```python
from build123d import *

# Parameters (mm, degrees)
BOSS_EXTRUDE1_DEPTH = 2
BOSS_EXTRUDE2_DEPTH = 60
CUT_EXTRUDE1_REACH  = 109.268
SKETCH2_R           = 11
SKETCH2_R_2         = 2.75
SKETCH3_R           = 2
CUT_EXTRUDE2_DEPTH  = 3
FILLET1_R           = 4


with BuildPart() as part:
    # Sketch1 → Boss-Extrude1 (new body)
    with BuildSketch(Plane(origin=(0, 0, 0), x_dir=(0, 0, -1), z_dir=(1, 0, 0))):
        Polygon((12.587763003, 38.086063364), (80, 3), (3.839824897, 3), align=None)
        Polygon((9.676875824, 38.811829051), (12.587763003, 38.086063364), (3.839824897, 3), (80, 3), (80, 0), (0, 0), align=None)
    extrude(amount=-BOSS_EXTRUDE1_DEPTH)

    # Sketch1<3> → Boss-Extrude2 (add)
    with BuildSketch(Plane(origin=(0, 0, 0), x_dir=(0, 0, -1), z_dir=(1, 0, 0))):
        Polygon((9.676875824, 38.811829051), (12.587763003, 38.086063364), (3.839824897, 3), (80, 3), (80, 0), (0, 0), align=None)
    extrude(amount=-BOSS_EXTRUDE2_DEPTH)

    # Sketch2 → Cut-Extrude1 (cut, up to next)
    with BuildSketch(Plane(origin=(0, 0, 0), x_dir=(1, 0, 0), z_dir=(0, 0.24192189559967164, 0.9702957262759956)), mode=Mode.PRIVATE) as cut_extrude1_sk1:
        with Locations(Location((-30, 20, 0), (0, 0, 270))):
            Circle(SKETCH2_R)
    cut_extrude1_tool1 = extrude(cut_extrude1_sk1.sketch, amount=-CUT_EXTRUDE1_REACH, mode=Mode.PRIVATE) & part.part
    # Sketch2 → Cut-Extrude1 (cut, up to next)
    with BuildSketch(Plane(origin=(0, 0, 0), x_dir=(1, 0, 0), z_dir=(0, 0.24192189559967164, 0.9702957262759956)), mode=Mode.PRIVATE) as cut_extrude1_sk2:
        with Locations(Location((-50, 20, 0), (0, 0, 270))):
            Circle(SKETCH2_R_2)
    cut_extrude1_tool2 = extrude(cut_extrude1_sk2.sketch, amount=-CUT_EXTRUDE1_REACH, mode=Mode.PRIVATE) & part.part
    # Sketch2 → Cut-Extrude1 (cut, up to next)
    with BuildSketch(Plane(origin=(0, 0, 0), x_dir=(1, 0, 0), z_dir=(0, 0.24192189559967164, 0.9702957262759956)), mode=Mode.PRIVATE) as cut_extrude1_sk3:
        with Locations(Location((-10, 20, 0), (0, 0, 90))):
            Circle(SKETCH2_R_2)
    cut_extrude1_tool3 = extrude(cut_extrude1_sk3.sketch, amount=-CUT_EXTRUDE1_REACH, mode=Mode.PRIVATE) & part.part
    add(cut_extrude1_tool1.solids().sort_by_distance((-30, 19.405915, -4.838438))[0], mode=Mode.SUBTRACT)
    add(cut_extrude1_tool2.solids().sort_by_distance((-50, 19.405915, -4.838438))[0], mode=Mode.SUBTRACT)
    add(cut_extrude1_tool3.solids().sort_by_distance((-10, 19.405915, -4.838438))[0], mode=Mode.SUBTRACT)

    # Sketch3 → Cut-Extrude2 (cut)
    with BuildSketch(Plane.XZ):
        with Locations(Location((-55, -33, 0), (0, 0, 270))):
            Circle(SKETCH3_R)
        with Locations(Location((-47, -33, 0), (0, 0, 270))):
            Circle(SKETCH3_R)
        with Locations(Location((-39, -33, 0), (0, 0, 270))):
            Circle(SKETCH3_R)
        with Locations(Location((-31, -33, 0), (0, 0, 270))):
            Circle(SKETCH3_R)
        with Locations(Location((-23, -33, 0), (0, 0, 270))):
            Circle(SKETCH3_R)
        with Locations(Location((-15, -33, 0), (0, 0, 270))):
            Circle(SKETCH3_R)
        with Locations(Location((-47, -41, 0), (0, 0, 270))):
            Circle(SKETCH3_R)
        with Locations(Location((-39, -41, 0), (0, 0, 270))):
            Circle(SKETCH3_R)
        with Locations(Location((-31, -41, 0), (0, 0, 270))):
            Circle(SKETCH3_R)
        with Locations(Location((-23, -41, 0), (0, 0, 270))):
            Circle(SKETCH3_R)
        with Locations(Location((-15, -41, 0), (0, 0, 270))):
            Circle(SKETCH3_R)
        with Locations(Location((-47, -49, 0), (0, 0, 270))):
            Circle(SKETCH3_R)
        with Locations(Location((-39, -49, 0), (0, 0, 270))):
            Circle(SKETCH3_R)
        with Locations(Location((-31, -49, 0), (0, 0, 270))):
            Circle(SKETCH3_R)
        with Locations(Location((-23, -49, 0), (0, 0, 270))):
            Circle(SKETCH3_R)
        with Locations(Location((-15, -49, 0), (0, 0, 270))):
            Circle(SKETCH3_R)
        with Locations(Location((-47, -57, 0), (0, 0, 270))):
            Circle(SKETCH3_R)
        with Locations(Location((-39, -57, 0), (0, 0, 270))):
            Circle(SKETCH3_R)
        with Locations(Location((-31, -57, 0), (0, 0, 270))):
            Circle(SKETCH3_R)
        with Locations(Location((-23, -57, 0), (0, 0, 270))):
            Circle(SKETCH3_R)
        with Locations(Location((-15, -57, 0), (0, 0, 270))):
            Circle(SKETCH3_R)
        with Locations(Location((-47, -65, 0), (0, 0, 270))):
            Circle(SKETCH3_R)
        with Locations(Location((-39, -65, 0), (0, 0, 270))):
            Circle(SKETCH3_R)
        with Locations(Location((-31, -65, 0), (0, 0, 270))):
            Circle(SKETCH3_R)
        with Locations(Location((-23, -65, 0), (0, 0, 270))):
            Circle(SKETCH3_R)
        with Locations(Location((-15, -65, 0), (0, 0, 270))):
            Circle(SKETCH3_R)
        with Locations(Location((-47, -73, 0), (0, 0, 270))):
            Circle(SKETCH3_R)
        with Locations(Location((-39, -73, 0), (0, 0, 270))):
            Circle(SKETCH3_R)
        with Locations(Location((-31, -73, 0), (0, 0, 270))):
            Circle(SKETCH3_R)
        with Locations(Location((-23, -73, 0), (0, 0, 270))):
            Circle(SKETCH3_R)
        with Locations(Location((-15, -73, 0), (0, 0, 270))):
            Circle(SKETCH3_R)
        with Locations(Location((-55, -41, 0), (0, 0, 270))):
            Circle(SKETCH3_R)
        with Locations(Location((-55, -49, 0), (0, 0, 270))):
            Circle(SKETCH3_R)
        with Locations(Location((-55, -57, 0), (0, 0, 270))):
            Circle(SKETCH3_R)
        with Locations(Location((-55, -65, 0), (0, 0, 270))):
            Circle(SKETCH3_R)
        with Locations(Location((-55, -73, 0), (0, 0, 270))):
            Circle(SKETCH3_R)
    extrude(amount=-CUT_EXTRUDE2_DEPTH, mode=Mode.SUBTRACT)

    # Fillet1
    fillet1_edges = [part.edges().sort_by_distance(p)[0] for p in [
        (-31, 3, -3.839824897),
    ]]
    fillet(fillet1_edges, radius=FILLET1_R)


solid = part.part
```
Design review of the part built by this model. Coordinates are the model's own, in mm. A direction names the side the tool comes from. Coordinates: 2 decimals unless noted, no trailing zeros. Order: outer loops, then holes, each group sorted by start corner. A loop starts at its lowest first (then second) coordinate and runs counter-clockwise, first axis right, second up. Notation, with made-up numbers: M 52.5,23.5 L 109.5,23.5 A18 cw 109.5,45.5 Z; hole C 5,13.5 d10. An arc over 180 degrees is marked long. Answer as a JSON object with one key per item and string values. Group by question number.
1) For pin 1 (6.5 mm diameter, centred on x = -39, z = -73, fed in from +Y); pin 2 (12 mm diameter, centred on x = -47.5, y = 16, fed in from -Z); pin 3 (10 mm diameter, centred on y = 14, z = -29, fed in from -X), all flat-tipped, find the tip position at first contact; note any pin that passes through.
2) Add section A-A, the plane x = -15. Count the separate pieces of the cut face and the enclosed holes in it, then the cut area to 3 significant figures.
3) Tool access review of faces 1 (the cylindrical face through (-53, 1, -57)), 2 (the flat face through (-30.594, 29.931, -10.554)): name each direction out of +Z, -Z, +X, -X, +Y, -Y from which nothing blocks a thin tool from reaching the whole face with its end or side.
4) Wall thickness on L1, parallel to X at y = 12, z = -22.5; L2, parallel to Y at x = -6, z = -19.5; L3, parallel to X at y = 25.5, z = -7.5: over which ranges is each line inside the solid? List them lowest first.
5) Add section D-D, the plane y = 31. Write out the cut boundary in (x, z), then the cut area to 3 significant figures.
6) Mouldability with a two-part tool opening along X and no side actions: class faces 3 (the cylindrical face through (-21, 1, -49)), 4 (the flat face through (-2, 13, -35)), 5 (the flat face through (-36, 0, -41)) as pulls with the +X half, pulls with the -X half, needs draft (parallel to the pull), parting line crosses it, or undercut.
Computed values:
{
 "1": {"pin 1": "stops at y = 3", "pin 2": "stops at z = -8.58", "pin 3": "stops at x = -2"},
 "2": {"separate pieces": "7", "enclosed holes": "0", "area": "282 mm^2"},
 "3": {"face 1": "+Y, -Y", "face 2": "-Z, -X"},
 "4": {"L1": "x = -2 to 0", "L2": "y = 0 to 3", "L3": "x = -60 to -38.83, -21.17 to 0"},
 "5": {"outline": "M -60,-10.82 L -2,-10.82 L -2,-26.2 L 0,-26.2 L 0,-7.73 L -60,-7.73 Z", "area": "216 mm^2"},
 "6": {"face 3": "undercut", "face 4": "pulls with the -X half", "face 5": "needs draft"}
}
